Design review of the part built by this model. Coordinates are the model's own, in mm. A direction names the side the tool comes from. Coordinates: 2 decimals unless noted, no trailing zeros. Loops run counter-clockwise (first coordinate to the right, second up) from the corner with the lowest first, then second, coordinate; pieces in that order, holes last. Notation, with made-up numbers: M 79,-14.5 L 108,-14.5 A20 ccw 108,21.5 Z; hole C 1,0 d1. An arc over 180 degrees is marked long. Put each result on its own line as item: value. Start each with the question number.
(1) The part is to be moulded in two halves that separate along X. For faces 3 (the cylindrical face through (18.02, 262.05, -36.49)), 4 (the cylindrical face through (1.61, 35.2, -15.27)), say which applies: +X half, -X half, draft (parallel to the pull), parting line (faces both ways), or undercut.
(2) Take a section at A-A, the plane z = -11. Give the boundary of the cut face in (x, y) (3 decimals).
(3) Take a section at C-C, the plane y = 88.9. Count the separate pieces of the cut face and the enclosed holes in it, then the cut area to 3 significant figures.
(4) For faces 1 (the flat face through (34.925, 150, -19)), 2 (the cylindrical face through (18.02, 84.25, -1.57)), list the 3-axis set-ups (+Z, -Z, +X, -X, +Y, -Y) from which the entire face can be reached by the end or side of a thin tool; tool diameter is ignored.
(5) For probe 1 along X at (y, z) = (270, -15.5) (3 decimals); probe 2 along Z at (x, y) = (28.5, 144.5) (3 decimals); probe 3 along Z at (x, y) = (36, 161), list the stretches that pass through material, from the lowest coordinate up. Write a range as [from, to].
(6) Take a section at B-B, the plane y = 50. Give the boundary of the cut face in (x, z) (3 decimals).
```python
from build123d import *

# Parameters (mm, degrees)
SKETCH1_W           = 38.1
SKETCH1_H           = 38.1
SKETCH1_W_2         = 31.75
SKETCH1_H_2         = 31.75
BOSS_EXTRUDE1_DEPTH = 304.8
FILLET1_R           = 3.175
SKETCH2_R           = 4.7625
CUT_EXTRUDE1_DEPTH  = 310.525863217
SKETCH3_R           = 4.7625
CUT_EXTRUDE2_DEPTH  = 310.525863217


with BuildPart() as part:
    # Sketch1 → Boss-Extrude1 (new body)
    with BuildSketch(Plane(origin=(0, 0, 0), x_dir=(1, 0, 0), z_dir=(0, 1, 0))):
        with Locations((19.05, 19.05)):
            Rectangle(SKETCH1_W, SKETCH1_H)
        with Locations((19.05, 19.05)):
            Rectangle(SKETCH1_W_2, SKETCH1_H_2, mode=Mode.SUBTRACT)
    extrude(amount=BOSS_EXTRUDE1_DEPTH)

    # Fillet1
    fillet1_edges = [part.edges().sort_by_distance(p)[0] for p in [
        (3.175, 152.4, -34.925),
        (3.175, 152.4, -3.175),
        (34.925, 152.4, -3.175),
        (34.925, 152.4, -34.925),
        (0, 152.4, -38.1),
        (38.1, 152.4, -38.1),
        (38.1, 152.4, 0),
        (0, 152.4, 0),
    ]]
    fillet(fillet1_edges, radius=FILLET1_R)

    # Sketch2 → Cut-Extrude1 (cut, through all)
    with BuildSketch(Plane.XY):
        with Locations((19.05, 12.7)):
            Circle(SKETCH2_R)
        with Locations((19.05, 38.1)):
            Circle(SKETCH2_R)
        with Locations((19.05, 63.5)):
            Circle(SKETCH2_R)
        with Locations((19.05, 88.9)):
            Circle(SKETCH2_R)
        with Locations((19.05, 114.3)):
            Circle(SKETCH2_R)
        with Locations((19.05, 139.7)):
            Circle(SKETCH2_R)
        with Locations((19.05, 165.1)):
            Circle(SKETCH2_R)
        with Locations((19.05, 190.5)):
            Circle(SKETCH2_R)
        with Locations((19.05, 215.9)):
            Circle(SKETCH2_R)
        with Locations((19.05, 241.3)):
            Circle(SKETCH2_R)
        with Locations((19.05, 266.7)):
            Circle(SKETCH2_R)
        with Locations((19.05, 292.1)):
            Circle(SKETCH2_R)
    extrude(amount=-CUT_EXTRUDE1_DEPTH, mode=Mode.SUBTRACT)

    # Sketch3 → Cut-Extrude2 (cut, through all)
    with BuildSketch(Plane(origin=(38.1, 0, 0), x_dir=(0, 0, -1), z_dir=(1, 0, 0))):
        with Locations((19.05, 12.7)):
            Circle(SKETCH3_R)
        with Locations((19.05, 38.1)):
            Circle(SKETCH3_R)
        with Locations((19.05, 63.5)):
            Circle(SKETCH3_R)
        with Locations((19.05, 88.9)):
            Circle(SKETCH3_R)
        with Locations((19.05, 114.3)):
            Circle(SKETCH3_R)
        with Locations((19.05, 139.7)):
            Circle(SKETCH3_R)
        with Locations((19.05, 165.1)):
            Circle(SKETCH3_R)
        with Locations((19.05, 190.5)):
            Circle(SKETCH3_R)
        with Locations((19.05, 215.9)):
            Circle(SKETCH3_R)
        with Locations((19.05, 241.3)):
            Circle(SKETCH3_R)
        with Locations((19.05, 266.7)):
            Circle(SKETCH3_R)
        with Locations((19.05, 292.1)):
            Circle(SKETCH3_R)
    extrude(amount=-CUT_EXTRUDE2_DEPTH, mode=Mode.SUBTRACT)


solid = part.part
```
Computed values:
1. face 3: undercut
1. face 4: draft
2. outline: M 0,0 L 3.175,0 L 3.175,304.8 L 0,304.8 Z; M 34.925,0 L 38.1,0 L 38.1,304.8 L 34.925,304.8 Z
3. separate pieces: 4
3. enclosed holes: 0
3. area: 323 mm^2
4. face 1: +Y, -Y
4. face 2: +Z, -Z
5. probe 1: x = [0, 3.175], [34.925, 38.1]
5. probe 2: z = [-38.1, -34.925], [-3.175, 0]
5. probe 3: z = [-37.91, -21.47], [-16.63, -0.19]
6. outline: M 0,-34.925 A3.175 ccw 3.175,-38.1 L 34.925,-38.1 A3.175 ccw 38.1,-34.925 L 38.1,-3.175 A3.175 ccw 34.925,0 L 3.175,0 A3.175 ccw 0,-3.175 Z; hole M 3.175,-31.75 A3.175 ccw 6.35,-34.925 L 31.75,-34.925 A3.175 ccw 34.925,-31.75 L 34.925,-6.35 A3.175 ccw 31.75,-3.175 L 6.35,-3.175 A3.175 ccw 3.175,-6.35 Z
